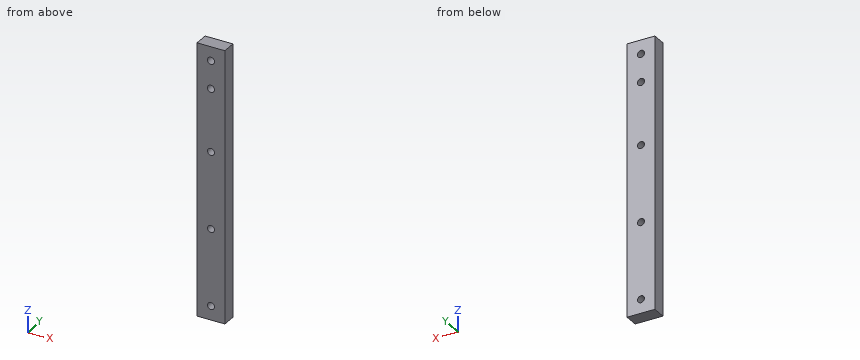
```python
from build123d import *

# Parameters (mm, degrees)
SKETCH1_W                   = 25.4
SKETCH1_H                   = 12.7
BOSS_EXTRUDE1_DEPTH         = 247.65
F_1_4_CLEARANCE_HOLE1_D     = 6.5278
F_1_4_0_25_DIAMETER_HOLE1_D = 6.35


with BuildPart() as part:
    # Sketch1 → Boss-Extrude1 (new body)
    with BuildSketch(Plane.XY):
        Rectangle(SKETCH1_W, SKETCH1_H)
    extrude(amount=BOSS_EXTRUDE1_DEPTH)

    # 1/4 Clearance Hole1 (through all)
    with Locations(Plane(origin=(0, 6.35, 0), x_dir=(1, 0, 0), z_dir=(0, 1, 0))):
        with Locations((0, -234.95), (0, -209.55)):
            Hole(F_1_4_CLEARANCE_HOLE1_D / 2)

    # 1/4 (0.25) Diameter Hole1 (through all)
    with Locations(Plane(origin=(0, 6.35, 0), x_dir=(1, 0, 0), z_dir=(0, 1, 0))):
        with Locations((0, -82.55), (0, -12.7), (0, -152.4)):
            Hole(F_1_4_0_25_DIAMETER_HOLE1_D / 2)


solid = part.part
```
Could you check a few things on this model? Use its own coordinates, in mm. Coordinates: 2 decimals unless noted, no trailing zeros. Loops run counter-clockwise (first coordinate to the right, second up) from the corner with the lowest first, then second, coordinate; pieces in that order, holes last.
1) Imagine slicing it at A-A (z = 152.4). List the corners of the cut face in (x, y) for me (3 decimals), and give its area (3 significant figures).
Reported:
outline: (-12.7, -6.35) - (-3.175, -6.35) - (-3.175, 6.35) - (-12.7, 6.35) - close; (3.175, -6.35) - (12.7, -6.35) - (12.7, 6.35) - (3.175, 6.35) - close
area: 242 mm2
2) Imagine slicing it at B-B (x = 0). List the corners of the cut face in (y, z) for me (3 decimals).
Reported:
outline: (-6.35, 0) - (6.35, 0) - (6.35, 9.525) - (-6.35, 9.525) - close; (-6.35, 15.875) - (6.35, 15.875) - (6.35, 79.375) - (-6.35, 79.375) - close; (-6.35, 85.725) - (6.35, 85.725) - (6.35, 149.225) - (-6.35, 149.225) - close; (-6.35, 155.575) - (6.35, 155.575) - (6.35, 206.286) - (-6.35, 206.286) - close; (-6.35, 212.814) - (6.35, 212.814) - (6.35, 231.686) - (-6.35, 231.686) - close; (-6.35, 238.214) - (6.35, 238.214) - (6.35, 247.65) - (-6.35, 247.65) - close
3) Imagine slicing it at D-D (z = 234.95). List the corners of the cut face in (x, y) for me.
Reported:
outline: (-12.7, -6.35) - (-3.26, -6.35) - (-3.26, 6.35) - (-12.7, 6.35) - close; (3.26, -6.35) - (12.7, -6.35) - (12.7, 6.35) - (3.26, 6.35) - close
4) Please list where these lines run through material, in increasing order: line 1 along Z through (x, y) = (0, -1.5) (3 decimals); line 2 along X through (y, z) = (2, 234.95); line 3 along X through (y, z) = (-1.25, 82.55) (3 decimals).
Reported:
line 1: z = 0 to 9.525, 15.875 to 79.375, 85.725 to 149.225, 155.575 to 206.286, 212.814 to 231.686, 238.214 to 247.65
line 2: x = -12.7 to -3.26, 3.26 to 12.7
line 3: x = -12.7 to -3.175, 3.175 to 12.7
5) Imagine slicing it at C-C (y = 3.25). List the corners of the cut face in (x, z) for me (3 decimals), and give its area (3 significant figures).
Reported:
outline: (-12.7, 0) - (12.7, 0) - (12.7, 247.65) - (-12.7, 247.65) - close; hole circle Ø6.528 at (0, 209.55); hole circle Ø6.528 at (0, 234.95); hole circle Ø6.35 at (0, 12.7); hole circle Ø6.35 at (0, 82.55); hole circle Ø6.35 at (0, 152.4)
area: 6,130 mm2
